Read the model definition and answer for the solid it produces. Units are mm, in the model's axes. A direction names the side the tool comes from. Give positions to 0.01 mm unless a question says otherwise; leave off trailing zeros. Order: outer loops, then holes, each group sorted by start corner. A loop starts at its lowest first (then second) coordinate and runs counter-clockwise, first axis right, second up. Notation, with made-up numbers: (32, 38) - (36, 38) arc R20 cw to (36, 71) - close; hole circle Ø4 at (-19.5, 3.25). An arc over 180 degrees is marked (long way). Write each question's results on one line, items separated by ' | '. Start each with the question number.
Q1. Find section B-B on x = 0. Give the vertices of the cut face in (y, z).
Q2. Find section C-C on z = 3.25. Count the separate pieces of the cut face and the enclosed holes in it, and give its area (3 significant figures).
Q3. Find section A-A on y = 7.5. Give the vertices of the cut face in (x, z).
Q4. For a pull along X with two mould halves and no side action, classify faces 1 (the face through (39.9, -24.4, 3.5)), 2 (the face through (24.81, -0.99, 3.55)), 3 (the face through (-22.5, 6, 3)) as +X half, -X half, draft (parallel to the pull), parting line (faces both ways), or undercut.
Q5. Flat-ended cylindrical pins translate along their axes: P1, Ø15.5, axis at x = 0, y = 7.5, coming from the +Z side; P2, Ø4, axis at x = -19, z = 5.5, coming from the -Y side; P3, Ø4, axis at y = -6.5, z = 3.5, coming from the -X side; P4, Ø4, axis at y = -10.5, z = 4, coming from the -X side. Find the tip coordinate at first contact, or state that the pin passes through.
Q6. A tool of negligible diameter and unlimited length cuts with its end or side. For faces 4 (the face through (35.29, -3.83, 3.45)), 5 (the face through (39.215, -12.018, 3.549)), 6 (the face through (19.231, -29.176, 3.451)), from which of +Z, -Z, +X, -X, +Y, -Y can it reach the whole face along a straight path? Write none if from no direction.
Q7. Find section D-D on x = -36.5. Give the vertices of the cut face in (y, z), and give its area (3 significant figures).
Q8. Find the intervals of material crossed by line 1 along X through (y, z) = (7.5, 2.25); line 2 along Y through (x, z) = (43, 3.5); line 3 along X through (y, z) = (-11.5, 3), in increasing order. Write a range as from..to.
from build123d import *

# Parameters (mm, degrees)
BOSS_EXTRUDE1_DEPTH     = 7
CUT_EXTRUDE1_DEPTH      = 10
CUT_EXTRUDE2_DEPTH      = 10
SKETCH6_W               = 67.896181325
SKETCH6_H               = 26.410991635
CUT_EXTRUDE3_DEPTH      = 8
CUT_EXTRUDE3_DEPTH_BACK = 1
FILLET1_R               = 8


with BuildPart() as part:
    # Sketch2 → Boss-Extrude1 (new body)
    with BuildSketch(Plane.XY):
        with BuildLine():
            Line((47.778278861, -11.389322146), (22.444705062, 3.947002617))
            Line((22.444705062, 3.947002617), (22.444705062, 13.423543635))
            ThreePointArc((22.444705062, 13.423543635), (0.788712907, 37.486172016), (-22.5, 15))
            Line((-22.5, 15), (-22.5, 3.913528416))
            Line((-22.5, 3.913528416), (-47.778278861, -11.389322146))
            Line((-47.778278861, -11.389322146), (-32.24208854, -37.05304733))
            Line((-32.24208854, -37.05304733), (-6.578363356, -21.516857009))
            ThreePointArc((-6.578363356, -21.516857009), (0, -22.5), (6.578363356, -21.516857009))
            Line((6.578363356, -21.516857009), (32.24208854, -37.05304733))
            Line((32.24208854, -37.05304733), (47.778278861, -11.389322146))
        make_face()
    extrude(amount=BOSS_EXTRUDE1_DEPTH)

    # Sketch4 → Cut-Extrude1 (cut)
    with BuildSketch(Plane.XY.offset(7)):
        Polygon((-43.658287311, -12.402075633), (-40.236457286, -10.33058359), (-38.164965243, -13.752413614), (-41.586795268, -15.823905657), align=None)
        Polygon((-23.127307163, 0.026876624), (-26.549137188, -2.044615419), (-24.477645145, -5.466445443), (-21.055815121, -3.3949534), align=None)
        Polygon((-31.229335054, -32.93305578), (-33.300827097, -29.511225755), (-29.878997072, -27.439733712), (-27.807505029, -30.861563737), align=None)
        Polygon((-10.698354907, -20.504103523), (-12.76984695, -17.082273498), (-16.191676974, -19.153765541), (-14.120184931, -22.575595566), align=None)
        Polygon((23.127307163, 0.026876624), (26.549137188, -2.044615419), (24.477645145, -5.466445443), (21.055815121, -3.3949534), align=None)
        Polygon((43.658287311, -12.402075633), (40.236457286, -10.33058359), (38.164965243, -13.752413614), (41.586795268, -15.823905657), align=None)
        Polygon((31.229335054, -32.93305578), (33.300827097, -29.511225755), (29.878997072, -27.439733712), (27.807505029, -30.861563737), align=None)
        Polygon((10.698354907, -20.504103523), (12.76984695, -17.082273498), (16.191676974, -19.153765541), (14.120184931, -22.575595566), align=None)
    extrude(amount=-CUT_EXTRUDE1_DEPTH, mode=Mode.SUBTRACT)

    # Sketch5 → Cut-Extrude2 (cut)
    with BuildSketch(Plane.XY.offset(7)):
        with BuildLine():
            Line((5.454356057, 10), (-5.454356057, 10))
            ThreePointArc((-5.454356057, 10), (0, 1.5), (5.454356057, 10))
        make_face()
    extrude(amount=-CUT_EXTRUDE2_DEPTH, mode=Mode.SUBTRACT)

    # Sketch6 → Cut-Extrude3 (cut, two sides)
    with BuildSketch(Plane.XY) as cut_extrude3_sk:
        with Locations((-0.747480896, 30.205495818)):
            Rectangle(SKETCH6_W, SKETCH6_H)
    extrude(amount=CUT_EXTRUDE3_DEPTH, mode=Mode.SUBTRACT)
    extrude(cut_extrude3_sk.sketch, amount=-CUT_EXTRUDE3_DEPTH_BACK, mode=Mode.SUBTRACT)

    # Fillet1
    fillet1_edges = [part.edges().sort_by_distance(p)[0] for p in [
        (22.410934831, 17, 3.5),
        (-22.410934831, 17, 3.5),
    ]]
    fillet(fillet1_edges, radius=FILLET1_R)


solid = part.part
Working result:
1) outline: (-22.5, 0) - (1.5, 0) - (1.5, 7) - (-22.5, 7) - close; (10, 0) - (17, 0) - (17, 7) - (10, 7) - close
2) separate pieces: 1 | enclosed holes: 9 | area: 2,880 mm²
3) outline: (-22.5, 0) - (-6, 0) - (-6, 7) - (-22.5, 7) - close; (6, 0) - (22.44, 0) - (22.44, 7) - (6, 7) - close
4) face 1: +X half | face 2: undercut | face 3: -X half
5) P1: z = 7 | P2: y = -30.25 | P3: x = -43.01 | P4: x = -47.78
6) face 4: +Z, -Z, +X, +Y | face 5: +Z, -Z | face 6: +Z, -Z, -Y
7) outline: (-30.02, 0) - (-4.56, 0) - (-4.56, 7) - (-30.02, 7) - close | area: 178 mm²
8) line 1: -22.5..-6, 6..22.44 | line 2: -19.28..-13.49, -12..-8.5 | line 3: -47.71..-42.17, -39.53..39.53, 42.17..47.71
